from build123d import *

# Parameters (mm, degrees)
F0_W      = 100
F0_H      = 100
F1_DEPTH  = 4
F3_DEPTH  = 4
F5_DEPTH  = 25
F6_R      = 0.5
F8_R      = 0.5
F9_R      = 0.5
F10_R     = 0.5
F11_R     = 3.75
F11_R_2   = 2.5
F12_DEPTH = 2.5


with BuildPart() as f1:
    # F0 (on Top) → F1 (new body)
    with BuildSketch(Plane.XY):
        with Locations((-18.7459290028, -1.397985096)):
            Rectangle(F0_W, F0_H)
    extrude(amount=F1_DEPTH)

    # F4 (on face) → F5 (cut)
    with BuildSketch(Plane(origin=(0, 0, 0), x_dir=(1, 0, 0), z_dir=(0, 0, -1))):
        Polygon((-23.8459290028, -48.602014904), (-18.7459290028, -48.602014904), (-18.7459290028, -43.552014904), (-13.7459290028, -43.602014904), (-13.7459290028, -38.502014904), (-23.8459290028, -38.502014904), align=None)
        Polygon((-68.7459290028, 5.1), (-68.7459290028, 0), (-63.7459290028, 0), (-63.7459290028, -5), (-58.6459290028, -5), (-58.6459290028, 5.1), align=None)
    extrude(amount=-F5_DEPTH, mode=Mode.SUBTRACT)

    # F6
    f6_edges = [f1.edges().sort_by_distance(p)[0] for p in [
        (31.254071, -51.397985, 2),
        (31.254071, 48.602015, 2),
        (-68.745929, 48.602015, 2),
        (-68.745929, -51.397985, 2),
    ]]
    fillet(f6_edges, radius=F6_R)


with BuildPart() as f3:
    # F2 (on face) → F3 (new body)
    with BuildSketch(Plane(origin=(0, 0, 0), x_dir=(1, 0, 0), z_dir=(0, 0, -1))):
        Polygon((-23.7459290028, 51.397985096), (-18.7459290028, 51.397985096), (-18.7459290028, 56.397985096), (-13.7459290028, 56.397985096), (-13.7459290028, 61.397985096), (-23.7459290028, 61.397985096), align=None)
    extrude(amount=-F3_DEPTH)


with BuildPart() as f3b:
    # F2 (on face) → F3, piece 2 (new body)
    with BuildSketch(Plane(origin=(0, 0, 0), x_dir=(1, 0, 0), z_dir=(0, 0, -1))):
        Polygon((41.2540709972, 5), (31.2540709972, 5), (31.2540709972, 0), (36.2540709972, 0), (36.2540709972, -5), (41.2540709972, -5), align=None)
    extrude(amount=-F3_DEPTH)


with BuildPart() as f3_1:
    add(f3.part)

    # F7: union F1, F3b
    add(f1.part)
    add(f3b.part)

    # F8
    f8_edges = [f3_1.edges().sort_by_distance(p)[0] for p in [
        (-23.745929, -51.397985, 2),
        (-18.745929, -51.397985, 2),
        (-13.745929, -61.397985, 2),
        (-13.745929, -56.397985, 2),
        (-18.745929, -56.397985, 2),
        (-23.745929, -61.397985, 2),
        (31.254071, -5, 2),
        (41.254071, -5, 2),
        (41.254071, 5, 2),
        (36.254071, 5, 2),
        (36.254071, 0, 2),
        (31.254071, 0, 2),
        (-23.845929, 38.502015, 2),
        (-13.745929, 38.502015, 2),
        (-18.745929, 48.602015, 2),
        (-18.745929, 43.552015, 2),
        (-23.845929, 48.602015, 2),
        (-13.745929, 43.602015, 2),
    ]]
    fillet(f8_edges, radius=F8_R)

    # F9
    f9_edges = [f3_1.edges().sort_by_distance(p)[0] for p in [
        (-58.645929, 5, 2),
        (-68.745929, 0, 2),
    ]]
    fillet(f9_edges, radius=F9_R)

    # F10
    f10_edges = [f3_1.edges().sort_by_distance(p)[0] for p in [
        (-63.745929, 0, 2),
        (-63.745929, 5, 2),
        (-58.645929, -5.1, 2),
        (-68.745929, -5.1, 2),
    ]]
    fillet(f10_edges, radius=F10_R)

    # F11 (on face) → F12 (join)
    with BuildSketch(Plane.XY.offset(4)):
        with Locations((-63.7459290028, 43.602014904)):
            Circle(F11_R)
        with Locations((-63.7459290028, 43.602014904)):
            Circle(F11_R_2, mode=Mode.SUBTRACT)
        with Locations((26.2540709972, 43.602014904)):
            Circle(F11_R)
        with Locations((26.2540709972, 43.602014904)):
            Circle(F11_R_2, mode=Mode.SUBTRACT)
        with Locations((26.2540709972, -46.397985096)):
            Circle(F11_R)
        with Locations((26.2540709972, -46.397985096)):
            Circle(F11_R_2, mode=Mode.SUBTRACT)
        with Locations((-63.7459290028, -46.397985096)):
            Circle(F11_R)
        with Locations((-63.7459290028, -46.397985096)):
            Circle(F11_R_2, mode=Mode.SUBTRACT)
    extrude(amount=F12_DEPTH)


solid = f3_1.part
Can you work these out from the model? Positions are in its coordinate system, mm. A direction names the side the tool comes from. Coordinates: 2 decimals unless noted, no trailing zeros. Loops run counter-clockwise (first coordinate to the right, second up) from the corner with the lowest first, then second, coordinate; pieces in that order, holes last. Notation, with made-up numbers: (-4, -27.75) - (47, -27.75) arc R13 cw to (47, -10.75) - close; hole circle Ø3 at (37, -25.5). An arc over 180 degrees is marked (long way). Put each result on its own line as item: value. Start each with the question number.
Item 1: Which directions (+Z, -Z, +X, -X, +Y, -Y) give clear straight access to the entire face, cutting with the end or side of a thin tool? Please do faces 1 (the face through (-63.746, 2, 2)), 2 (the face through (-64, 44, 4)), 3 (the face through (-19, -61.398, 2)), 4 (the face through (-23.846, 43, 2)), 5 (the face through (-47, 48.602, 2)).
Item 2: Suppose I cut it at D-D (y = 34). Please give me the cut outline in (x, z).
Item 3: For pin 1 (3 mm diameter, centred on x = 37.5, z = 2, fed in from -Y); pin 2 (10 mm diameter, centred on x = 8.5, y = -43, fed in from +Z); pin 3 (2 mm diameter, centred on y = 15, z = 3, fed in from +X), each with a flat end and sliding along its axis, tell me the tip position at first contact or that it passes through.
Item 4: If I drill on line 1 along Y through (x, z) = (-17.5, 1); line 2 along Z through (x, y) = (16, -0.5); line 3 along Y through (x, z) = (13.5, 0.75), over which ranges is the centre line in solid material (lowest first)?
Item 5: Suppose I cut it at B-B (z = 5.25). Please give me the cut outline in (x, y), and give its area (3 significant figures).
Item 6: Suppose I cut it at C-C (x = 33.5). Please give me the cut outline in (y, z).
Item 7: Suppose I cut it at A-A (y = 3). Please give me the cut outline in (x, z), and give its area (3 significant figures).
Item 8: If we mould it in two halves opening along Y, with no side actions, what happens to faces 6 (the face through (39, 5, 2)), 7 (the face through (-58.646, 0, 2)), 8 (the face through (-23.746, -56, 2)), 9 (the face through (-64, -46, 4))? For each: +Y half, -Y half, draft (parallel to the pull), parting line (faces both ways), or undercut.
Here are the results:
1. face 1: +Z, -Z
1. face 2: +Z
1. face 3: +Z, -Z, +X, -X, -Y
1. face 4: +Z, -Z, +Y
1. face 5: +Z, -Z, +X, -X, +Y
2. outline: (-68.75, 0) - (31.25, 0) - (31.25, 4) - (-68.75, 4) - close
3. pin 1: y = -5
3. pin 2: z = 4
3. pin 3: x = 31.25
4. line 1: -61.4 to -56.4, -51.4 to 38.5, 43.56 to 48.6
4. line 2: 0 to 4
4. line 3: -51.4 to 48.6
5. outline: circle Ø7.5 at (-63.75, -46.4); circle Ø7.5 at (-63.75, 43.6); circle Ø7.5 at (26.25, -46.4); circle Ø7.5 at (26.25, 43.6); hole circle Ø5 at (-63.75, -46.4); hole circle Ø5 at (-63.75, 43.6); hole circle Ø5 at (26.25, -46.4); hole circle Ø5 at (26.25, 43.6)
5. area: 98.2 mm²
6. outline: (-5, 0) - (0, 0) - (0, 4) - (-5, 4) - close
7. outline: (-68.75, 0) - (-63.75, 0) - (-63.75, 4) - (-68.75, 4) - close; (-58.65, 0) - (31.25, 0) - (31.25, 4) - (-58.65, 4) - close; (36.25, 0) - (41.25, 0) - (41.25, 4) - (36.25, 4) - close
7. area: 400 mm²
8. face 6: +Y half
8. face 7: undercut
8. face 8: draft
8. face 9: undercut
